Autodesk Fusion 360 part; units mm, degrees
sketch "Sketch1" plane through (0, 0, 0) normal (0, 0, 1) x (1, 0, 0)
  line L0 (285.2, -291.299) -> (-285.2, -291.299)
  line L1 (-285.2, -291.299) -> (-285.2, 291.299)
  line L2 (-285.2, 291.299) -> (285.2, 291.299)
  line L3 (285.2, 291.299) -> (285.2, -291.299)
  line L4 (285.2, -291.299) -> (-285.2, 291.299) construction
  line L5 (-285.2, -291.299) -> (285.2, 291.299) construction
  line L6 (-262.35, 291.299) -> (-262.35, -291.299) construction
  circle A0 centre (-262.35, 280.639) radius 2
  circle A1 centre (-262.35, 266.5) radius 2
  circle A2 centre (-262.35, -280.639) radius 2
  circle A3 centre (-262.35, -266.5) radius 2
  line L7 (262.35, 291.299) -> (262.35, -291.299) construction
  circle A4 centre (262.35, 280.639) radius 2
  circle A5 centre (262.35, 266.5) radius 2
  circle A6 centre (262.35, -280.639) radius 2
  circle A7 centre (262.35, -266.5) radius 2
  line L8 (-262.35, -266.5) -> (262.35, -266.5) construction
  circle A8 centre (0, -273.16) radius 2
  line L9 (0, -291.299) -> (0, 291.299) construction
  circle A9 centre (0, 273.16) radius 2
  circle A10 centre (0, 287.299) radius 2
  circle A11 centre (0, -287.299) radius 2
  line L10 (200, 225) -> (-200, 225)
  line L11 (-200, 225) -> (-200, -225)
  line L12 (-200, -225) -> (200, -225)
  line L13 (200, -225) -> (200, 225)
  line L14 (200, 225) -> (-200, -225) construction
  line L15 (-200, 225) -> (200, -225) construction
  line L16 (-290.2, 296.299) -> (290.2, 296.299)
  line L17 (290.2, 296.299) -> (290.2, -296.299)
  line L18 (290.2, -296.299) -> (-290.2, -296.299)
  line L19 (-290.2, -296.299) -> (-290.2, 296.299)
  circle A12 centre (280.2, 101.299) radius 2
  circle A13 centre (280.2, -101.299) radius 2
  circle A14 centre (-280.2, -101.299) radius 2
  circle A15 centre (-280.2, 101.299) radius 2
  line L20 (-304.8, -372.499) -> (304.8, -372.499) construction
  line L21 (304.8, -372.499) -> (304.8, 541.901) construction
  line L22 (304.8, 541.901) -> (-304.8, 541.901) construction
  line L23 (-304.8, 541.901) -> (-304.8, -372.499) construction
  line L24 (0, -372.499) -> (0, -296.299) construction
  line L25 (-262.35, 266.5) -> (262.35, 266.5) construction
  line L26 (262.35, -280.639) -> (-262.35, -280.639) construction
  line L27 (262.35, 280.639) -> (-262.35, 280.639) construction
  dimension "d1" = 570.4
  dimension "d2" = 582.598
  dimension "d3" = 22.85
  dimension "d4" = 4
  dimension "d6" = 4
  dimension "d8" = 4
  dimension "d9" = 4
  dimension "d12" = 22.85
  dimension "d13" = 4
  dimension "d14" = 4
  dimension "d17" = 4
  dimension "d18" = 4
  dimension "d21" = 4
  dimension "d22" = 4
  dimension "d23" = 4
  dimension "d24" = 4
  dimension "d28" = 450
  dimension "d29" = 400
  dimension "d30" = 5
  dimension "d31" = 5
  dimension "d32" = 5
  dimension "d33" = 5
  dimension "d37" = 4
  dimension "d38" = 4
  dimension "d39" = 4
  dimension "d40" = 4
  dimension "d41" = 190
  dimension "d42" = 190
  dimension "d43" = 5
  dimension "d44" = 5
  dimension "d45" = 190
  dimension "d46" = 190
  dimension "d47" = 5
  dimension "d49" = 5
  dimension "d51" = 609.6
  dimension "d52" = 76.2
  dimension "d53" = 914.4
  dimension "d54" = 24.799
  dimension "d55" = 24.799
  dimension "d56" = 10.66
  dimension "d57" = 10.66
  dimension "d61" = 4
  dimension "d62" = 14.139
  dimension "d63" = 14.139
  dimension "d64" = 4
extrude "Extrude1" add sketch "Sketch1" along normal blind 5 contours L0 L1 L2 L3 | L16 L17 L18 L19 makes body 1
fillet "Fillet1" radius 20 4 edges at (-200, -225, 2.5) (200, -225, 2.5) (200, 225, 2.5) (-200, 225, 2.5) on bodies 1
copy_body "Body->Comp1" bodies 1 removing the originals makes body 2 in component "Front Panel"
component "Front Panel" placed x (1, 0, 0) y (0, 1, 0) z (0, 0, 1) at (0, 0, 0)
equation "d1 = XRailLength + 220.4 mm"
equation "d2 = PrintHeight + 282.598 mm"
equation "d28 = PrintHeight + 150 mm"
equation "d29 = XRailLength + 50 mm"
equation "d30 = WallThickness"
equation "d31 = WallThickness"
equation "d32 = WallThickness"
equation "d33 = WallThickness"
equation "WallThickness = 5 mm"
equation "XRailLength = 350 mm"
equation "PrintHeight = 300 mm"
For this review, take the finished solid that the model builds, in its own axes (mm). A direction names the side the tool comes from. Give positions to 0.01 mm unless a question says otherwise; leave off trailing zeros. Loops run counter-clockwise (first coordinate to the right, second up) from the corner with the lowest first, then second, coordinate; pieces in that order, holes last.
Item 1: Tool access review of faces 3 (the cylindrical face through (193.986, -219.297, 2.535)), 4 (the flat face through (254, 4, 0)): name each direction out of +Z, -Z, +X, -X, +Y, -Y from which nothing blocks a thin tool from reaching the whole face with its end or side.
Item 2: Draft analysis for pull direction Y (two halves, no side actions). For faces 1 (the cylindrical face through (194.297, 218.986, 2.535)), 2 (the flat face through (254, 4, 5)), state which applies: +Y half, -Y half, draft (parallel to the pull), parting line (faces both ways), or undercut.
Item 3: For line 1 along Y through (x, z) = (-263, 2.8); line 2 along X through (y, z) = (-266.5, 2.8); line 3 along Y through (x, z) = (262.35, 3.3), list the stretches that pass through material, from the lowest coordinate up.
Item 4: Take a section at C-C, the plane z = 1.9. Give the number of separate pieces and of enclosed holes in the cut face, and give its area (3 significant figures).
Item 5: Take a section at B-B, the plane x = 143. State the section outline as (y, z) points, and give its area (3 significant figures).
Item 6: Insertion check: pin 1 (3.5 mm diameter, centred on x = -262.35, y = -280.639, fed in from +Z). The pin has a flat end and moves straight along its axis. Give the tip position at first contact, or say it passes through.
Item 7: Take a section at A-A, the plane y = 145.5. State the section outline as (x, z) points.
Calculated:
1. face 3: +Z, -Z
1. face 4: -Z, +X, -X, +Y, -Y
2. face 1: undercut
2. face 2: draft
3. line 1: y = -296.3 to -282.53, -278.75 to -268.39, -264.61 to 264.61, 268.39 to 278.75, 282.53 to 296.3
3. line 2: x = -290.2 to -264.35, -260.35 to 260.35, 264.35 to 290.2
3. line 3: y = -296.3 to -282.64, -278.64 to -268.5, -264.5 to 264.5, 268.5 to 278.64, 282.64 to 296.3
4. separate pieces: 1
4. enclosed holes: 17
4. area: 164,000 mm2
5. outline: (-296.3, 0) - (-225, 0) - (-225, 5) - (-296.3, 5) - close; (225, 0) - (296.3, 0) - (296.3, 5) - (225, 5) - close
5. area: 713 mm2
6. pin 1: passes through
7. outline: (-290.2, 0) - (-200, 0) - (-200, 5) - (-290.2, 5) - close; (200, 0) - (290.2, 0) - (290.2, 5) - (200, 5) - close
